Source: CAD feature listing. Evaluate the final solid. Frame: model axes, mm. Face numbers are marked on the shaded views. A direction names the side the tool comes from. Coordinates: 2 decimals unless noted, no trailing zeros. Loops run counter-clockwise (first coordinate to the right, second up) from the corner with the lowest first, then second, coordinate; pieces in that order, holes last.
from build123d import *

# Parameters (mm, degrees)
SKETCH1_R           = 12.065
BOSS_EXTRUDE1_DEPTH = 12.7
SKETCH2_R           = 1.27
BOSS_EXTRUDE2_DEPTH = 6.35
SKETCH4_W           = 5.04217838
SKETCH4_H           = 7.772020178
CUT_EXTRUDE1_DEPTH  = 3.81
CHAMFER1_SIZE       = 0.508


with BuildPart() as part:
    # Sketch1 → Boss-Extrude1 (new body)
    with BuildSketch(Plane(origin=(0, 0, 0), x_dir=(0, 0, -1), z_dir=(1, 0, 0))):
        Circle(SKETCH1_R)
    extrude(amount=BOSS_EXTRUDE1_DEPTH)

    # Sketch2 → Boss-Extrude2 (add)
    with BuildSketch(Plane(origin=(12.7, 0, 0), x_dir=(0, 0, -1), z_dir=(1, 0, 0))):
        Circle(SKETCH2_R)
    extrude(amount=BOSS_EXTRUDE2_DEPTH)

    # Sketch4 → Cut-Extrude1 (cut)
    with BuildSketch(Plane.ZY):
        with Locations((-11.192351372, 0.27298418)):
            Rectangle(SKETCH4_W, SKETCH4_H)
    extrude(amount=-CUT_EXTRUDE1_DEPTH, mode=Mode.SUBTRACT)

    # Chamfer1
    chamfer1_edges = [part.edges().sort_by_distance(p)[0] for p in [
        (0, -0.288360149, 12.061553525),
        (12.7, 0, 12.065),
    ]]
    chamfer(chamfer1_edges, length=CHAMFER1_SIZE)


solid = part.part
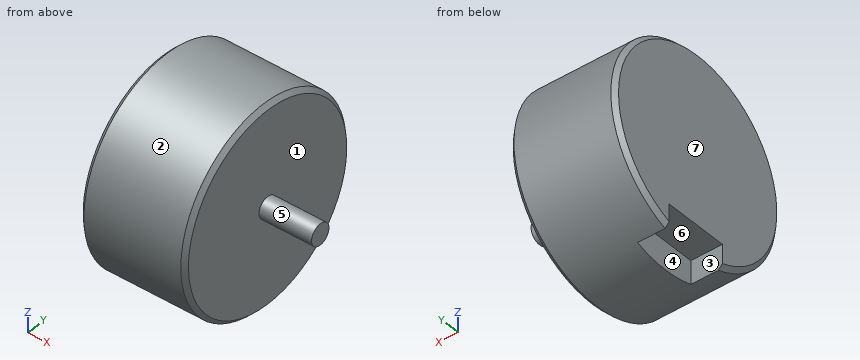
Q1. Draft query along Y for the marked faces 1, 2, 3 and 4. Return one class per face: +Y half, -Y half, draft (parallel to the pull), parting line (faces both ways), or undercut.
Q2. Access query for the marked faces 5, 6 and 7. Directions: +Z, -Z, +X, -X, +Y, -Y. A direction counts if a zero-diameter tool reaches every point of the face in a straight line with its end or side. Return the directions, or none.
Q3. Section B-B, the plane z = 0. Return the cut outline in (x, y) (3 decimals).
Q4. Section A-A, the plane y = 0. Return the cut outline in (x, z) (3 decimals).
Q5. Section D-D, the plane x = 9. Return the cut outline in (y, z) (3 decimals).
Q6. Section C-C, the plane x = 1.5. Return the cut outline in (y, z) (1 decimal), plus the area to 3 significant figures.
Q7. Contact query for flat-ended pins moving along their axis: pin 1 Ø8 at (x, z) = (13.5, 1.5) entering from -Y (3 decimals); pin 2 Ø5 at (x, z) = (14, 9) entering from +Y; pin 3 Ø2 at (x, z) = (3, -10) entering from -Y; pin 4 Ø8 at (y, z) = (-7.5, -8.5) entering from +X. Output: stop coordinate, or through.
Q8. Line query: line 1 along X through (y, z) = (10, -2); line 2 along X through (y, z) = (3, -9.75); line 3 along Y through (x, z) = (10.75, 2.75). Output: solid intervals per line, ascending.
Derived:
1. face 1: draft
1. face 2: parting line
1. face 3: undercut
1. face 4: undercut
2. face 5: +X
2. face 6: -Z, -X
2. face 7: +Z, -Z, -X, +Y, -Y
3. outline: (0, -11.557) - (0.508, -12.065) - (12.192, -12.065) - (12.7, -11.557) - (12.7, -1.27) - (19.05, -1.27) - (19.05, 1.27) - (12.7, 1.27) - (12.7, 11.557) - (12.192, 12.065) - (0.508, 12.065) - (0, 11.557) - close
4. outline: (0, -8.671) - (3.81, -8.671) - (3.81, -12.065) - (12.192, -12.065) - (12.7, -11.557) - (12.7, -1.27) - (19.05, -1.27) - (19.05, 1.27) - (12.7, 1.27) - (12.7, 11.557) - (12.192, 12.065) - (0.508, 12.065) - (0, 11.557) - close
5. outline: circle Ø24.13 at (0, 0)
6. outline: (-3.6, -11.5) - (-3.6, -8.7) - (4.2, -8.7) - (4.2, -11.3) arc R12.1 ccw (long way) to start
6. area: 433 mm2
7. pin 1: stops at y = -12.065
7. pin 2: stops at y = 9.63
7. pin 3: stops at y = -8.04
7. pin 4: stops at x = 12.7
8. line 1: x = 0 to 12.7
8. line 2: x = 3.81 to 12.7
8. line 3: y = -11.75 to 11.75
